from build123d import *

# Parameters (mm, degrees)
SKETCH1_W               = 66
SKETCH1_H               = 4
BOSS_EXTRUDE1_DEPTH     = 7
SKETCH2_R               = 1.65
CUT_EXTRUDE1_DEPTH      = 67.49060084
SKETCH3_W               = 5
SKETCH3_H               = 3.5
BOSS_EXTRUDE2_DEPTH     = 12
SKETCH4_W               = 5
SKETCH4_H               = 5
BOSS_EXTRUDE3_DEPTH     = 6
SKETCH5_W               = 4
SKETCH5_H               = 7
BOSS_EXTRUDE4_DEPTH     = 50
SKETCH7_W               = 5
SKETCH7_H               = 12
BOSS_EXTRUDE5_DEPTH     = 3.5
FILLET1_R               = 2
FILLET2_R               = 2
SKETCH8_W               = 4
SKETCH8_H               = 7
BOSS_EXTRUDE6_DEPTH     = 8.3
SKETCH9_W               = 4
SKETCH9_H               = 7
BOSS_EXTRUDE7_DEPTH     = 12
CUT_EXTRUDE2_DEPTH      = 117.828934772
CUT_EXTRUDE2_DEPTH_BACK = 117.828934772
SKETCH6_R               = 1.45
FILLET3_R               = 2
FILLET4_R               = 5
FILLET5_R               = 2


with BuildPart() as part:
    # Sketch1 → Boss-Extrude1 (new body)
    with BuildSketch(Plane(origin=(0, 0, 0), x_dir=(1, 0, 0), z_dir=(0, 1, 0))):
        with Locations((33, -2)):
            Rectangle(SKETCH1_W, SKETCH1_H)
    extrude(amount=BOSS_EXTRUDE1_DEPTH)

    # Sketch2 → Cut-Extrude1 (cut, through all)
    with BuildSketch(Plane.XY.offset(4)):
        with Locations((33, 3.5)):
            Circle(SKETCH2_R)
    extrude(amount=-CUT_EXTRUDE1_DEPTH, mode=Mode.SUBTRACT)

    # Sketch3 → Boss-Extrude2 (add)
    with BuildSketch(Plane(origin=(0, 0, 0), x_dir=(-1, 0, 0), z_dir=(0, 0, -1))):
        with Locations((-63.5, 1.75)):
            Rectangle(SKETCH3_W, SKETCH3_H)
        with Locations((-2.5, 1.75)):
            Rectangle(SKETCH3_W, SKETCH3_H)
    extrude(amount=BOSS_EXTRUDE2_DEPTH)

    # Sketch4 → Boss-Extrude3 (add)
    with BuildSketch(Plane(origin=(0, 0, 0), x_dir=(-1, 0, 0), z_dir=(0, -1, 0))):
        with Locations((-63.5, 9.5)):
            Rectangle(SKETCH4_W, SKETCH4_H)
        with Locations((-2.5, 9.5)):
            Rectangle(SKETCH4_W, SKETCH4_H)
    extrude(amount=BOSS_EXTRUDE3_DEPTH)

    # Sketch5 → Boss-Extrude4 (add)
    with BuildSketch(Plane(origin=(66, 0, 0), x_dir=(0, 0, -1), z_dir=(1, 0, 0))):
        with Locations((-2, 3.5)):
            Rectangle(SKETCH5_W, SKETCH5_H)
    extrude(amount=BOSS_EXTRUDE4_DEPTH)

    # Sketch7 → Boss-Extrude5 (add)
    with BuildSketch(Plane(origin=(0, 3.5, 0), x_dir=(1, 0, 0), z_dir=(0, 1, 0))):
        with Locations((63.5, 6)):
            Rectangle(SKETCH7_W, SKETCH7_H)
        with Locations((2.5, 6)):
            Rectangle(SKETCH7_W, SKETCH7_H)
    extrude(amount=BOSS_EXTRUDE5_DEPTH)

    # Fillet1
    fillet1_edges = [part.edges().sort_by_distance(p)[0] for p in [
        (66, -6, -9.5),
        (63.5, -6, -7),
        (61, -6, -9.5),
        (63.5, -6, -12),
        (5, -6, -9.5),
        (2.5, -6, -7),
        (0, -6, -9.5),
        (2.5, -6, -12),
    ]]
    fillet(fillet1_edges, radius=FILLET1_R)

    # Fillet2
    fillet2_edges = [part.edges().sort_by_distance(p)[0] for p in [
        (61, 3.5, 0),
        (5, 3.5, 0),
        (63.5, 0, -7),
        (2.5, 0, -7),
        (66, 3.5, 0),
        (116, 0, 2),
        (116, 7, 2),
        (0, 3.5, 4),
        (63.5, 7, -12),
        (2.5, 7, -12),
    ]]
    fillet(fillet2_edges, radius=FILLET2_R)

    # Sketch8 → Boss-Extrude6 (add)
    with BuildSketch(Plane(origin=(0, 0, 0), x_dir=(-1, 0, 0), z_dir=(0, 0, -1))):
        with Locations((-102, 3.5)):
            Rectangle(SKETCH8_W, SKETCH8_H)
    extrude(amount=BOSS_EXTRUDE6_DEPTH)

    # Sketch9 → Boss-Extrude7 (add)
    with BuildSketch(Plane(origin=(104, 0, 0), x_dir=(0, 0, -1), z_dir=(1, 0, 0))):
        with Locations((6.3, 3.5)):
            Rectangle(SKETCH9_W, SKETCH9_H)
    extrude(amount=BOSS_EXTRUDE7_DEPTH)

    # Sketch6 → Cut-Extrude2 (cut, two sides: drawn at the far end of the back side and taken through both)
    with BuildSketch(Plane(origin=(0, 0, 0), x_dir=(-1, 0, 0), z_dir=(0, 0, -1)).offset(-CUT_EXTRUDE2_DEPTH_BACK)):
        with Locations((-110, 3.5)):
            Circle(SKETCH6_R)
    extrude(amount=CUT_EXTRUDE2_DEPTH + CUT_EXTRUDE2_DEPTH_BACK, mode=Mode.SUBTRACT)

    # Fillet3
    fillet3_edges = [part.edges().sort_by_distance(p)[0] for p in [
        (116, 7, -6.3),
        (116, 0, -6.3),
    ]]
    fillet(fillet3_edges, radius=FILLET3_R)

    # Fillet4
    fillet4_edges = [part.edges().sort_by_distance(p)[0] for p in [
        (100, 3.5, 0),
    ]]
    fillet(fillet4_edges, radius=FILLET4_R)

    # Fillet5
    fillet5_edges = [part.edges().sort_by_distance(p)[0] for p in [
        (100, 3.5, -8.3),
    ]]
    fillet(fillet5_edges, radius=FILLET5_R)


solid = part.part
Read the model definition and answer for the solid it produces. Units are mm, in the model's axes. A direction names the side the tool comes from. Round coordinates to 2 decimals unless told otherwise and drop trailing zeros. Loops run counter-clockwise (first coordinate to the right, second up) from the corner with the lowest first, then second, coordinate; pieces in that order, holes last.
Q1. Section B-B on x = 110 is taken. Write down the section's boundary in (y, z).
Q2. Each of these flat-tipped pins is pushed along its axis until it touches: pin 1 (3.5 mm diameter, centred on x = 28, y = 2, fed in from -Z); pin 2 (5 mm diameter, centred on x = 100.5, z = -1.5, fed in from -Y); pin 3 (2.5 mm diameter, centred on x = 33, y = 3.5, fed in from +Z); pin 4 (1.6 mm diameter, centred on x = 1.5, y = -3.5, fed in from +Z). Where does it stop, or does it pass through?
Q3. Section D-D on x = 97 is taken. Write down the section's boundary in (y, z).
Q4. Section A-A on x = 33 is taken. Write down the section's boundary in (y, z), and give its area (3 significant figures).
Q5. Which of the six approach directions +Z, -Z, +X, -X, +Y, -Y give full straight-line access (tool end or side, diameter ignored) to faces 1 (the face through (3, -3, -7)), 2 (the face through (104, 3, -2)), 3 (the face through (107, 3, -8.3))?
Q6. Section C-C on y = 3.5 is taken. Give the number of separate pieces and of enclosed holes in the cut face, and give its area (3 significant figures).
Q7. Consider probe 1 along X at (y, z) = (1.75, -6.5); probe 2 along Y at (x, z) = (110, -6.25); probe 3 along X at (y, z) = (3.5, -6.5). Determine where each line is inside the solid, lowest interval first.
Q8. Determine the mould class of faces 4 (the face through (116, 4, -6)), 5 (the face through (66.57, 3.45, -0.6)), 6 (the face through (2.54, 6.43, -11.4)), 7 (the face through (100.57, 3.55, -7.7)) for opening direction X: released by +X, released by -X, zero draft, split by the parting line, or undercut.
Output:
1. outline: (0, -8.3) - (2.05, -8.3) - (2.05, -4.3) - (0, -4.3) - close; (0, 0) - (2.05, 0) - (2.05, 4) - (0, 4) - close; (4.95, -8.3) - (7, -8.3) - (7, -4.3) - (4.95, -4.3) - close; (4.95, 0) - (7, 0) - (7, 4) - (4.95, 4) - close
2. pin 1: stops at z = 0
2. pin 2: stops at y = 0
2. pin 3: passes through
2. pin 4: stops at z = -7
3. outline: (0, -0.42) - (7, -0.42) - (7, 4) - (0, 4) - close
4. outline: (0, 0) - (1.85, 0) - (1.85, 4) - (0, 4) - close; (5.15, 0) - (7, 0) - (7, 4) - (5.15, 4) - close
4. area: 14.8 mm2
5. face 1: +Z, +X, -X, -Y
5. face 2: +X, +Y, -Y
5. face 3: -Z, +X, +Y, -Y
6. separate pieces: 4
6. enclosed holes: 0
6. area: 635 mm2
7. probe 1: x = 0 to 5, 61 to 66, 100.01 to 115.98
7. probe 2: y = 0 to 2.05, 4.95 to 7
7. probe 3: x = 0 to 5, 61 to 66, 100.01 to 108.55, 111.45 to 116
8. face 4: released by +X
8. face 5: undercut
8. face 6: zero draft
8. face 7: undercut
